Source: CAD feature listing. Evaluate the final solid. Frame: model axes, mm. Face numbers are marked on the shaded views. A direction names the side the tool comes from. Round coordinates to 2 decimals unless told otherwise and drop trailing zeros. Order: outer loops, then holes, each group sorted by start corner. A loop starts at its lowest first (then second) coordinate and runs counter-clockwise, first axis right, second up. Notation, with made-up numbers: M 30,87 L 73,87 A16 cw 73,105 Z; hole C 7,31.5 d2. An arc over 180 degrees is marked long. Answer as CSV lines item,"result". Start each with the question number.
Item 1: Section query A-A on x = 95. Return the cut outline in (y, z), plus the area to 3 significant figures.
Item 2: Set-up query: the marked faces 4, 5, 6, 7 and 8. Return all of +Z, -Z, +X, -X, +Y, -Y with unobstructed straight access to the full face (end or side cutting, diameter ignored); none if empty.
Item 3: Section query B-B on y = 39. Return the cut outline in (x, z), plus the area to 3 significant figures.
Item 4: Section query C-C on z = 3.5. Return the cut outline in (x, y), plus the area to 3 significant figures.
Item 5: First-contact query: P1, Ø4, axis at x = 103.5, y = 16, coming from the +Z side; P2, Ø2, axis at x = 88.5, z = -27.5, coming from the -Y side; P3, Ø15, axis at x = 97, y = 44.5, coming from the -Z side. Flat tips, straight axial feed; report the tip coordinate or a pass-through.
Item 6: Pull-direction query (Y, two-part tool) for the marked faces 1, 2 and 3; classes: +Y half, -Y half, draft (parallel to the pull), parting line (faces both ways), or undercut.
Item 7: Line query: line 1 (Z direction, x = 120, y = 43.5); line 2 (Z direction, x = 111, y = -16.5); line 3 (Y direction, x = 123, z = -26). Output: solid intervals per line, ascending. Write a range as [from, to].
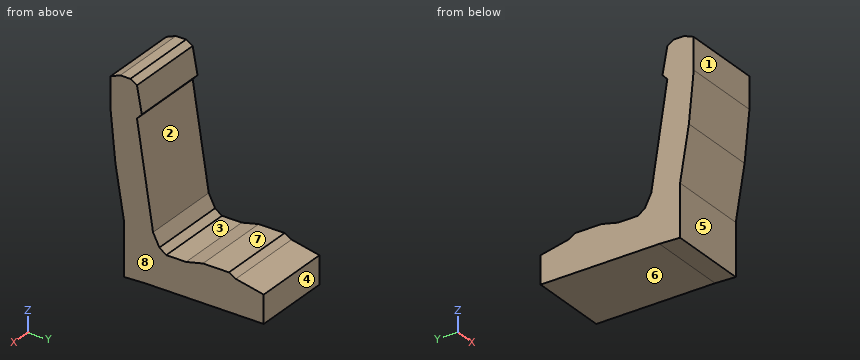
from build123d import *

# Parameters (mm, degrees)
F1_DEPTH = 127
F2_DEPTH = 76.2


with BuildPart() as f1:
    # F0 (on Right) → F1 (new body)
    with BuildSketch(Plane.YZ):
        Polygon((52.6268968752, -31.8920984864), (48.25777933, -29.3743014336), (40.0050003082, -29.3743014336), (31.7522212863, -29.3743014336), (21.0081070048, -31.9401308597), (8.4041413315, -31.9401308597), (4.0564504452, -28.8147889078), (0, -20.9816433489), (-10.2110654116, 43.9215712249), (-7.1337609552, 47.2786352038), (-10.2110654116, 63.7841969728), (-14.4073953852, 66.3019940257), (-20.8417680115, 66.3019940257), (-26.9963834435, 63.7841969728), (-26.9963834435, 43.9215712249), (-23.9190720022, 12.5889861956), (-18.3239672333, -20.9816433489), (-18.3239672333, -53.7130087614), (-5.1754736342, -53.1534962356), (70.3584477305, -53.1534962356), (70.3584477305, -45.0405962765), (70.3584477305, -35.5289168656), align=None)
    extrude(amount=F1_DEPTH)

    # F2 (cut): a face of the model
    f2_faces = [f1.faces().sort_by_distance(p)[0] for p in [
        (0, -23.9197614794, 28.4063291618),
    ]]
    extrude(f2_faces, amount=-F2_DEPTH, mode=Mode.SUBTRACT)


solid = f1.part
Results:
1,outline,"M -27,43.92 L -23.92,12.59 L -18.32,-20.98 L -18.32,-53.71 L -5.18,-53.15 L 70.36,-53.15 L 70.36,-35.53 L 52.63,-31.89 L 48.26,-29.37 L 31.75,-29.37 L 21.01,-31.94 L 8.4,-31.94 L 4.06,-28.81 L 0,-20.98 L -10.21,43.92 L -7.13,47.28 L -10.21,63.78 L -14.41,66.3 L -20.84,66.3 L -27,63.78 Z"
1,area,"3,720 mm^2"
2,face 4,"+Z, -Z, +X, -X, +Y"
2,face 5,"-Z, +X, -X, -Y"
2,face 6,"-Z, +X, -X, +Y"
2,face 7,"+Z, +X, -X, +Y"
2,face 8,"+Z, -Z, +X, +Y, -Y"
3,outline,"M 76.2,-53.15 L 127,-53.15 L 127,-29.37 L 76.2,-29.37 Z"
3,area,"1,210 mm^2"
4,outline,"M 76.2,-22.4 L 127,-22.4 L 127,-3.85 L 76.2,-3.85 Z"
4,area,"942 mm^2"
5,P1,"z = -31.94"
5,P2,"y = -18.32"
5,P3,"z = -53.15"
6,face 1,"-Y half"
6,face 2,"+Y half"
6,face 3,"undercut"
7,line 1,"[-53.15, -29.37]"
7,line 2,"[-53.64, 66.3]"
7,line 3,"[-18.32, 2.6]"
